Read the model definition and answer for the solid it produces. Units are mm, in the model's axes. Coordinates: 2 decimals unless noted, no trailing zeros. Loops run counter-clockwise (first coordinate to the right, second up) from the corner with the lowest first, then second, coordinate; pieces in that order, holes last.
from build123d import *

# Parameters (mm, degrees)
SKETCH1_R           = 40
BOSS_EXTRUDE1_DEPTH = 30
FILLET1_R           = 10
SKETCH2_R           = 2.5
CUT_EXTRUDE1_DEPTH  = 30


with BuildPart() as part:
    # Sketch1 → Boss-Extrude1 (new body)
    with BuildSketch(Plane.XY):
        Circle(SKETCH1_R)
    extrude(amount=BOSS_EXTRUDE1_DEPTH)

    # Fillet1
    fillet1_edges = [part.edges().sort_by_distance(p)[0] for p in [
        (-40, 0, 0),
        (-40, 0, 30),
    ]]
    fillet(fillet1_edges, radius=FILLET1_R)

    # Sketch2 → Cut-Extrude1 (cut)
    with BuildSketch(Plane.XY.offset(30)):
        Circle(SKETCH2_R)
    extrude(amount=-CUT_EXTRUDE1_DEPTH, mode=Mode.SUBTRACT)


solid = part.part
Q1. Straight lines are drawn through the part: probe 1 along Y at (x, z) = (0, 13.25); probe 2 along Y at (x, z) = (0, 22.75); probe 3 along X at (y, z) = (17.5, 6.5). For each, find the intervals that lie inside material, in ascending order.
Findings below:
probe 1: y = -40 to -2.5, 2.5 to 40
probe 2: y = -39.61 to -2.5, 2.5 to 39.61
probe 3: x = -35.26 to 35.26
Q2. A cutting plane is placed at D-D (z = 25.5). Give the vertices of the cut face in (x, y).
Findings below:
outline: circle Ø76.7 at (0, 0); hole circle Ø5 at (0, 0)
Q3. A cutting plane is placed at A-A (y = 0). Give the vertices of the cut face in (x, z).
Findings below:
outline: (-40, 10) arc R10 ccw to (-30, 0) - (-2.5, 0) - (-2.5, 30) - (-30, 30) arc R10 ccw to (-40, 20) - close; (2.5, 0) - (30, 0) arc R10 ccw to (40, 10) - (40, 20) arc R10 ccw to (30, 30) - (2.5, 30) - close
Q4. Flat-ended cylindrical pins translate along their axes: pin 1 Ø1 at (y, z) = (17, 24.5) entering from -X; pin 2 Ø10 at (x, y) = (-16, -26.5) entering from +Z; pin 3 Ø8 at (y, z) = (-22.5, 14) entering from +X; pin 4 Ø1.5 at (x, z) = (-27, 24) entering from +Y. Find the tip coordinate at first contact, or state that the pin passes through.
Findings below:
pin 1: stops at x = -35.38
pin 2: stops at z = 30
pin 3: stops at x = 35.46
pin 4: stops at y = 29.18
Q5. Determine the mould class of faces 1 (the face through (-8.67, -39.05, 14.93)), 2 (the face through (-0.54, -2.44, 15.21)), 3 (the face through (0, -6, 30)) for opening direction Y: +Y half, -Y half, draft (parallel to the pull), parting line (faces both ways), or undercut.
Findings below:
face 1: parting line
face 2: undercut
face 3: draft
Q6. A cutting plane is placed at C-C (z = 2). Give the vertices of the cut face in (x, y), then the cut area to 3 significant figures.
Findings below:
outline: circle Ø72 at (0, 0); hole circle Ø5 at (0, 0)
area: 4,050 mm2
